Input: dimensioned drawing with shaded views. Units: mm. Origin: part minimum x, y, z. Round coordinates to 2 decimals unless told otherwise and drop trailing zeros. Loops run counter-clockwise (first coordinate to the right, second up) from the corner with the lowest first, then second, coordinate; pieces in that order, holes last. Notation, with made-up numbers: (14.25, 70.5) -> (71.25, 70.5) arc R30 ccw to (71.25, 93.5) -> close; hole circle Ø10 at (79.5, 31). An arc over 180 degrees is marked (long way). Answer as a JSON object with one key per item and string values.
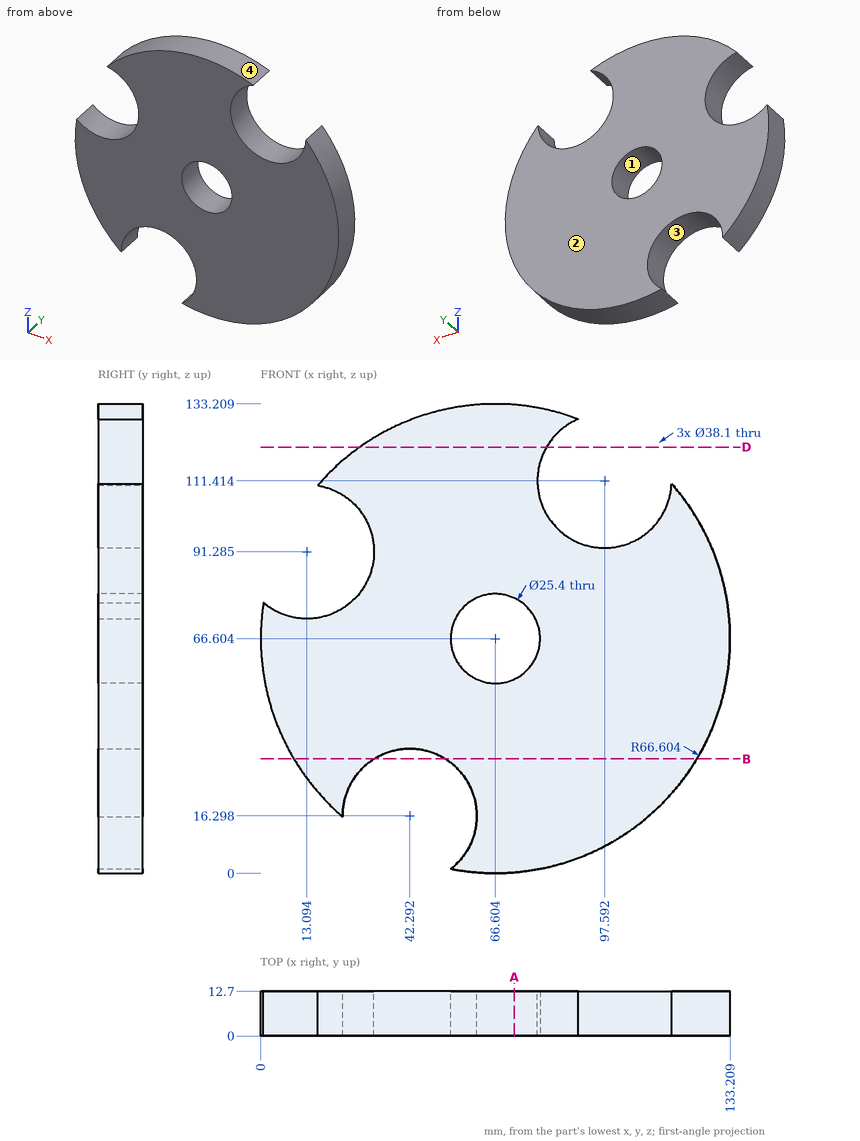
1) Draft query along X for the marked faces 1, 2, 3 and 4. Return one class per face: +X half, -X half, draft (parallel to the pull), parting line (faces both ways), or undercut.
Output:
{"face 1": "undercut", "face 2": "draft", "face 3": "undercut", "face 4": "parting line"}
2) Contact query for flat-ended pins moving along their axis: P1, Ø4, axis at x = 63.5, y = 6.5, coming from the +Z side; P2, Ø5, axis at y = 7.5, z = 14, coming from the +X side; P3, Ø4, axis at x = 78, y = 8.5, coming from the -Z side. Output: stop coordinate, or through.
Output:
{"P1": "stops at z = 133.2", "P2": "stops at x = 110.49", "P3": "stops at z = 0.67"}
3) Section D-D, the plane z = 121. Output: boundary loops of the cut face in (x, y).
Output:
{"outline": "(28.17, 0) -> (81.13, 0) -> (81.13, 12.7) -> (28.17, 12.7) -> close"}
4) Section A-A, the plane x = 72. Output: boundary loops of the cut face in (y, z).
Output:
{"outline": "(0, 0.22) -> (12.7, 0.22) -> (12.7, 55.11) -> (0, 55.11) -> close; (0, 78.1) -> (12.7, 78.1) -> (12.7, 132.99) -> (0, 132.99) -> close"}
5) Ray query, probe 1 along X at (y, z) = (11, 64.5) (1 decimal); probe 2 along X at (y, z) = (2.75, 55) (1 decimal); probe 3 along Z at (x, y) = (55.5, 11.25) (1 decimal). Return the intervals inside material, ascending.
Output:
{"probe 1": "x = 0 to 54.1, 79.1 to 133.2", "probe 2": "x = 1 to 61.4, 71.8 to 132.2", "probe 3": "z = 0.9 to 2.6, 30 to 60.4, 72.8 to 132.3"}
6) Section B-B, the plane z = 32.5. Output: boundary loops of the cut face in (x, y) (1 decimal), plus the area to 3 significant figures.
Output:
{"outline": "(9.4, 0) -> (32.3, 0) -> (32.3, 12.7) -> (9.4, 12.7) -> close; (52.3, 0) -> (123.8, 0) -> (123.8, 12.7) -> (52.3, 12.7) -> close", "area": "1,200 mm^2"}
